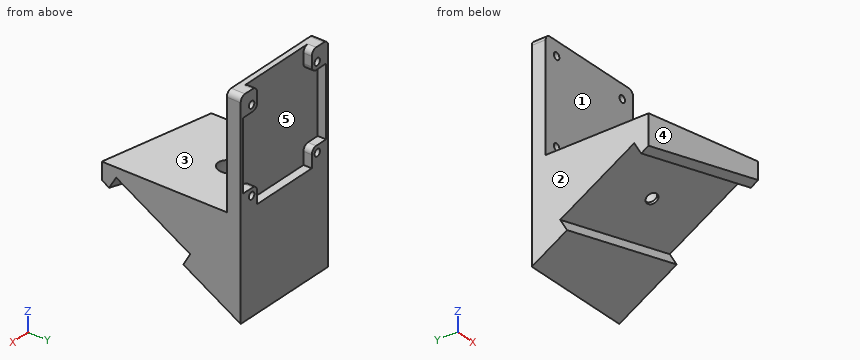
Autodesk Inventor part; units mm, degrees
ref_plane "Work Plane3" through (20, 15.5, 9.3468) normal (0, -0.5, -0.8660254) x (-1, 0, 0)
ref_plane "YZ Plane" through (0, 0, 0) normal (1, 0, 0) x (0, 1, 0)
ref_plane "XZ Plane" through (0, 0, 0) normal (0, 1, 0) x (-1, 0, 0)
sketch "Sketch1" plane through (0, 0, 0) normal (0, 1, 0) x (-1, 0, 0)
  line L0 (19, 19) -> (-19, 19) construction
  line L1 (-19, 19) -> (-19, -19) construction
  line L2 (-19, -19) -> (19, -19) construction
  line L3 (19, -19) -> (19, 19) construction
  line L4 (19, 19) -> (-19, -19) construction
  line L5 (-19, 19) -> (19, -19) construction
  circle A0 centre (15, -15) radius 1.25
  circle A1 centre (-15, -15) radius 1.25
  circle A2 centre (15, 15) radius 1.25
  circle A3 centre (-15, 15) radius 1.25
  line L6 (20, 20) -> (-20, 20)
  line L7 (-20, 20) -> (-20, -20)
  line L8 (-20, -20) -> (20, -20)
  line L9 (20, -20) -> (20, 20)
  line L10 (20, 20) -> (-20, -20) construction
  line L11 (-20, 20) -> (20, -20) construction
  point P0 (0, 0)
  dimension "d0" = 38
  dimension "d1" = 38
  dimension "d2" = 2.5
  dimension "d3" = 2.5
  dimension "d4" = 2.5
  dimension "d5" = 2.5
  dimension "d6" = 4
  dimension "d7" = 4
  dimension "d8" = 4
  dimension "d9" = 4
  dimension "d10" = 40
  dimension "d11" = 40
extrude "Extrusion1" add sketch "Sketch1" along normal blind 5
sketch "Sketch2" plane through (0, 5, 0) normal (0, 1, 0) x (1, 0, 0)
  line L0 (-12.5, 19) -> (-12.5, 12.5)
  line L1 (-12.5, 12.5) -> (-19, 12.5)
  line L2 (-19, 12.5) -> (-19, -12.5)
  line L3 (-20, 20) -> (-20, -20)
  line L4 (-19, -12.5) -> (-12.5, -12.5)
  line L5 (-12.5, -12.5) -> (-12.5, -20)
  line L6 (-12.5, -20) -> (12.5, -20)
  line L7 (12.5, -20) -> (12.5, -12.5)
  line L8 (12.5, -12.5) -> (19, -12.5)
  line L9 (19, -12.5) -> (19, 12.5)
  line L10 (19, 12.5) -> (12.5, 12.5)
  line L11 (12.5, 12.5) -> (12.5, 19)
  line L12 (12.5, 19) -> (-12.5, 19)
  point P0 (0, 0)
  dimension "d14" = 25
  dimension "d15" = 6.5
  dimension "d16" = 25
  dimension "d17" = 7.5
  dimension "d18" = 6.5
  dimension "d19" = 6.5
  dimension "d20" = 25
  dimension "d21" = 6.5
  dimension "d22" = 12.5
  dimension "d24" = 12.5
extrude "Extrusion2" cut sketch "Sketch2" against normal blind 3
sketch "Sketch3" plane through (0, 2, 0) normal (0, 1, 0) x (1, 0, 0)
  line L0 (12.5, -12.5) -> (12.5, -20)
  line L1 (-12.5, -20) -> (12.5, -20)
  line L2 (12.5, -20) -> (12.5, -16)
  line L3 (12.5, -16) -> (-12.5, -16)
  line L4 (-12.5, -16) -> (-12.5, -20)
  point P0 (0, 0)
  dimension "d27" = 4
extrude "Extrusion3" cut sketch "Sketch3" against normal through all
fillet "Fillet1" radius 2 10 edges at (-20, 2.5, -20) (20, 2.5, -20) (-20, 2.5, 20) (20, 2.5, 20) (-12.5, 3.5, -12.5) (12.5, 3.5, -12.5) (12.5, 3.5, 12.5) (-12.5, 3.5, 12.5) (-12.5, 2.5, 20) (12.5, 2.5, 20)
sketch "Sketch4" plane through (0, 0, 0) normal (0, -1, 0) x (1, 0, 0)
  line L0 (-20, -17.5) -> (20, -17.5)
  line L1 (20, -17.5) -> (20, 17.5)
  line L2 (20, 17.5) -> (-20, 17.5)
  line L3 (-20, 17.5) -> (-20, -17.5)
  line L4 (-20, -17.5) -> (20, 17.5) construction
  line L5 (20, -17.5) -> (-20, 17.5) construction
  point P0 (0, 0)
  dimension "d31" = 40
  dimension "d32" = 35
extrude "Extrusion4" add sketch "Sketch4" along normal blind 50
sketch "Sketch6" plane through (-20, 0, 17.5) normal (0, 0, 1) x (1, 0, 0)
  line L0 (40, 0) -> (40, -50)
  line L1 (40, -50) -> (0, -42.0435)
  line L2 (0, 0) -> (0, -50)
  line L3 (40, -50) -> (80.7836, -50) construction
  line L4 (0, -42.0435) -> (0, -50)
  line L5 (0, -50) -> (40, -50)
  point P0 (20, 0)
  dimension "d35" = 168.75
extrude "Extrusion5" cut sketch "Sketch6" against normal through all
sketch "Sketch7" plane through (20, 0, 17.5) normal (1, 0, 0) x (0, 0, 1)
  line L0 (-35, 0) -> (-35, 50)
  line L1 (-35, 0) -> (-6.1325, 50)
  line L2 (-35, 50) -> (0, 50)
  line L3 (-35, 0) -> (22.735, 0) construction
  line L4 (-6.1325, 50) -> (-35, 50)
  line L5 (-35, 50) -> (-35, 0)
  point P0 (-17.5, 0)
  dimension "d38" = 120
extrude "Extrusion6" cut sketch "Sketch7" against normal through all
sketch "Sketch17" plane through (20, 0, -17.5) normal (0, -0.5, -0.8660254) x (-1, 0, 0)
  line L0 (40, -48.5477) -> (0, -57.735) construction
  line L1 (40, 0) -> (40, -48.5477) construction
  line L2 (0, 0) -> (40, 0) construction
  line L3 (0, -57.735) -> (0, 0) construction
  line L4 (0, -54.6569) -> (40, -45.4695) construction
  line L5 (0, -23.8758) -> (40, -14.6884) construction
  line L6 (0, -54.6569) -> (40, -45.4695)
  line L7 (40, -14.6884) -> (0, -23.8758)
  line L8 (0, -23.8758) -> (0, -54.6569)
  line L9 (40, -45.4695) -> (40, -14.6884)
  point P0 (20, -8.75)
  dimension "d60" = 30
  dimension "d61" = 3
extrude "Extrusion9" cut sketch "Sketch17" against normal blind 5
sketch "Sketch18" plane through (20, 2.5, -13.1699) normal (0, -0.5, -0.8660254) x (-1, 0, 0)
  line L0 (40, -14.6884) -> (40, -45.4695) construction
  line L1 (0, -23.8758) -> (40, -14.6884) construction
  line L2 (0, -54.6569) -> (0, -23.8758) construction
  line L3 (40, -45.4695) -> (0, -54.6569) construction
  line L4 (0, -54.6569) -> (40, -14.6884) construction
  line L5 (0, -23.8758) -> (40, -45.4695) construction
  circle A0 centre (20, -34.6727) radius 2
  circle A1 centre (20, -34.6727) radius 4.6064
  point P0 (20, -8.75)
  dimension "d64" = 4
extrude "Extrusion11" cut sketch "Sketch18" against normal through all contours A0
ref_plane "Work Plane3" through (20, 15.5, 9.3468) normal (0, -0.5, -0.8660254) x (-1, 0, 0)
sketch "Sketch20" plane through (20, 15.5, 9.3468) normal (0, -0.5, -0.8660254) x (-1, 0, 0)
  circle A0 centre (20, -34.6727) radius 2
  circle A1 centre (20, -34.6727) radius 3.5
  point P0 (20, -8.75)
  dimension "d70" = 7
extrude "Extrusion12" cut sketch "Sketch20" along normal blind 25
sketch "Sketch21" plane through (-20, 0, 17.5) normal (0, 0, 1) x (1, 0, 0)
  line L0 (0, 0) -> (40, 0)
  line L1 (40, 0) -> (40, -5)
  line L2 (40, -5) -> (0, -5)
  line L3 (0, -5) -> (0, 0)
  point P0 (20, 0)
  dimension "d73" = 5
extrude "Extrusion13" add sketch "Sketch21" along normal blind 40
sketch "Sketch22" plane through (20, 0, -18) normal (1, 0, 0) x (0, 0, -1)
  line L0 (2, 0) -> (0, 0)
  line L1 (-38, 5) -> (-36, 5)
  line L2 (2, 0) -> (-38, 0)
  line L3 (-38, 0) -> (-38, 5)
  line L4 (-38, 5) -> (2, 5)
  line L5 (2, 5) -> (2, 0)
  point P0 (-18, 0)
extrude "Extrusion14" cut sketch "Sketch22" against normal through all
sketch "Sketch23" plane through (-20, 0, 57.5) normal (0, 1, 0) x (1, 0, 0)
  line L0 (40, 0) -> (0, 0) construction
  line L1 (20, 0) -> (20, 20) construction
  line L2 (39, 39) -> (1, 39) construction
  line L3 (1, 39) -> (1, 1) construction
  line L4 (1, 1) -> (39, 1) construction
  line L5 (39, 1) -> (39, 39) construction
  line L6 (39, 39) -> (1, 1) construction
  line L7 (1, 39) -> (39, 1) construction
  circle A0 centre (35, 5) radius 1.25
  line L8 (20, 20) -> (1, 20) construction
  circle A1 centre (5, 5) radius 1.25
  circle A2 centre (35, 35) radius 1.25
  circle A3 centre (5, 35) radius 1.25
  point P0 (20, 57.5)
  dimension "d78" = 20
  dimension "d79" = 38
  dimension "d80" = 38
  dimension "d81" = 4
  dimension "d82" = 2.5
extrude "Extrusion15" cut sketch "Sketch23" against normal through all
sketch "Sketch24" plane through (-20, 0, 57.5) normal (0, 1, 0) x (1, 0, 0)
  line L0 (1, 7.5) -> (7.5, 7.5)
  line L1 (7.5, 7.5) -> (7.5, 0)
  line L2 (7.5, 0) -> (32.5, 0)
  line L3 (32.5, 0) -> (32.5, 7.5)
  line L4 (32.5, 7.5) -> (39, 7.5)
  line L5 (39, 7.5) -> (39, 32.5)
  line L6 (39, 32.5) -> (32.5, 32.5)
  line L7 (32.5, 32.5) -> (32.5, 39)
  line L8 (32.5, 39) -> (7.5, 39)
  line L9 (7.5, 39) -> (7.5, 32.5)
  line L10 (7.5, 32.5) -> (1, 32.5)
  line L11 (1, 32.5) -> (1, 7.5)
  line L12 (0, 0) -> (40, 0) construction
  line L13 (0, 75) -> (0, 0)
  point P0 (20, 57.5)
  point P1 (39, 20)
  point P2 (20, 39)
  dimension "d85" = 6.5
  dimension "d86" = 25
  dimension "d87" = 6.5
  dimension "d88" = 25
  dimension "d90" = 7.5
  dimension "d91" = 25
  dimension "d92" = 6.5
  dimension "d93" = 20
  dimension "d94" = 7.5
  dimension "d95" = 6.5
  dimension "d96" = 20
extrude "Extrusion16" cut sketch "Sketch24" against normal blind 3
fillet "Fillet2" radius 2 8 edges at (-12.5, -1.5, 50) (-12.5, -1.5, 25) (12.5, -1.5, 25) (12.5, -1.5, 50) (12.5, -1.5, 57.5) (-12.5, -1.5, 57.5) (20, -2.5, 57.5) (-20, -2.5, 57.5)
properties part number "CameraMountM12v2"
Geometry: final body of the model. Coordinates: model frame, mm. Face numbers are marked on the shaded views. A direction names the side the tool comes from. Round coordinates to 2 decimals unless told otherwise and drop trailing zeros. Loops run counter-clockwise (first coordinate to the right, second up) from the corner with the lowest first, then second, coordinate; pieces in that order, holes last. Notation, with made-up numbers: (-3, 11.25) -> (15, 11.25) arc R4 cw to (15, 16.25) -> close; hole circle Ø3 at (-7.75, 50). An arc over 180 degrees is marked (long way). One line per question, with ' | ' between items. Start each with the question number.
1. Section D-D on y = -38. Output: boundary loops of the cut face in (x, z).
2. Section A-A on x = 1. Output: boundary loops of the cut face in (y, z).
3. Contact query for flat-ended pins moving along their axis: pin 1 (4 mm diameter, centred on x = 6, y = -27.5, fed in from +Z); pin 2 (1.5 mm diameter, centred on x = -6, y = -1, fed in from +Z); pin 3 (10 mm diameter, centred on x = 1.5, y = -15.5, fed in from -Z); pin 4 (1.5 mm diameter, centred on x = 15, z = 52.5, fed in from +Y). Output: stop coordinate, or through.
4. Mould query, pull axis Z, two halves, no side actions, for the marked faces 3, 4 and 5. Classes: pulls with the +Z half, pulls with the -Z half, needs draft (parallel to the pull), parting line crosses it, or undercut.
5. Line query: line 1 along X through (y, z) = (-3.9, 52.5); line 2 along X through (y, z) = (-1.05, 52.5); line 3 along X through (y, z) = (-1, 52). Output: solid intervals per line, ascending. Write a range as [from, to].
6. Set-up query: the marked faces 1 and 2. Return all of +Z, -Z, +X, -X, +Y, -Y with unobstructed straight access to the full face (end or side cutting, diameter ignored); none if empty.
7. Section B-B on z = 49. Output: boundary loops of the cut face in (x, y), and give its area (3 significant figures).
8. Section C-C on x = 11. Output: boundary loops of the cut face in (y, z), and give its area (3 significant figures).
Returned:
1) outline: (-20, 7.62) -> (-14.35, 10.22) -> (20, 10.22) -> (20, 17.5) -> (-20, 17.5) -> close
2) outline: (-46.22, 9.19) -> (-43.55, 7.65) -> (-41.05, 11.98) -> (-29.03, 5.03) -> (-28.53, 5.9) -> (-29.93, 6.71) -> (-23.7, 17.5) -> (-46.22, 17.5) -> close; (-26.03, 3.3) -> (-14.4, -3.41) -> (-16.9, -7.74) -> (0, -17.5) -> (0, 18.5) -> (-3, 18.5) -> (-3, 57.5) -> (-5, 57.5) -> (-5, 17.5) -> (-15.96, 17.5) -> (-24.12, 3.35) -> (-25.53, 4.16) -> close
3) pin 1: stops at z = 17.5 | pin 2: stops at z = 18.5 | pin 3: stops at z = -11.44 | pin 4: passes through
4) face 3: pulls with the +Z half | face 4: needs draft | face 5: undercut
5) line 1: x = [-20, -16.25], [-13.75, 13.75], [16.25, 20] | line 2: x = [-20, -16.25], [-13.75, -12.5], [12.5, 13.75], [16.25, 20] | line 3: x = [-20, -16.15], [-13.85, -12.5], [12.5, 13.85], [16.15, 20]
6) face 1: +Z, +X, -X, -Y | face 2: +Z, -Z, -X, +Y, -Y
7) outline: (-20, -5) -> (20, -5) -> (20, 0) -> (19, 0) -> (19, -3) -> (-19, -3) -> (-19, 0) -> (-20, 0) -> close | area: 86.0 mm2
8) outline: (-48.21, 10.33) -> (-45.54, 8.79) -> (-43.04, 13.13) -> (-16.39, -2.26) -> (-18.89, -6.6) -> (0, -17.5) -> (0, 18.5) -> (-3, 18.5) -> (-3, 57.5) -> (-5, 57.5) -> (-5, 17.5) -> (-48.21, 17.5) -> close | area: 945 mm2
